Could you check a few things on this model? Use its own coordinates, in mm. A direction names the side the tool comes from. Round coordinates to 2 decimals unless told otherwise and drop trailing zeros. Loops run counter-clockwise (first coordinate to the right, second up) from the corner with the lowest first, then second, coordinate; pieces in that order, holes last. Notation, with made-up numbers: (61, -23.5) - (99, -23.5) arc R19 ccw to (99, -8.5) - close; hole circle Ø11 at (84.25, 56.5). An arc over 180 degrees is marked (long way). Use one line per item in the form item = value.
Autodesk Fusion 360 part; units mm, degrees
sketch "Sketch1" plane through (0, 0, 0) normal (0, 0, 1) x (1, 0, 0)
  line L0 (0, 26.67) -> (-38.1, 26.67)
  line L1 (0, -26.67) -> (-38.1, -26.67)
  line L2 (-38.1, 24.257) -> (0, 24.257)
  line L3 (-38.1, -24.257) -> (0, -24.257)
  line L4 (-38.1, 26.67) -> (-38.1, 24.257)
  line L5 (-38.1, -24.257) -> (-38.1, -26.67)
  arc A0 (0, -26.67) -> (0, 26.67) centre (0, 0) ccw
  arc A1 (0, -24.257) -> (0, 24.257) centre (0, 0) ccw
  dimension "d1" = 53.34
  dimension "d2" = 48.514
  dimension "d3" = 38.1
  dimension "d4" = 38.1
extrude "Extrude1" add sketch "Sketch1" along normal blind 5
sketch "Sketch2" plane through (0, 0, 5) normal (0, 0, 1) x (-1, 0, 0)
  line L0 (38.1, 24.257) -> (38.1, 26.67)
  line L1 (38.1, 26.67) -> (0, 26.67)
  arc A0 (0, 26.67) -> (0, -26.67) centre (0, 0) ccw
  line L2 (0, -26.67) -> (38.1, -26.67)
  line L3 (38.1, -26.67) -> (38.1, -24.257)
  line L4 (38.1, -24.257) -> (0, -24.257)
  arc A1 (0, 24.257) -> (0, -24.257) centre (0, 0) ccw
  line L5 (0, 24.257) -> (38.1, 24.257)
  line L6 (38.1, -26.67) -> (38.1, 26.67)
extrude "Extrude2" add sketch "Sketch2" along normal blind 2.54
sketch "Sketch3" plane through (0, 0, 7.54) normal (0, 0, 1) x (-1, 0, 0)
  line L0 (38.1, -26.67) -> (38.1, 26.67)
  line L1 (38.1, 26.67) -> (0, 26.67)
  arc A0 (0, 26.67) -> (0, -26.67) centre (0, 0) ccw
  line L2 (0, -26.67) -> (38.1, -26.67)
  circle A1 centre (0, 0) radius 16.51
  dimension "d9" = 33.02
extrude "Extrude3" cut sketch "Sketch3" against normal through all contours A1
sketch "Sketch4" plane through (0, 0, 5) normal (0, 0, -1) x (1, 0, 0)
  circle A0 centre (0, 0) radius 16.51
  line L0 (0, 24.257) -> (-38.1, 24.257)
  line L1 (-38.1, 24.257) -> (-38.1, -24.257)
  line L2 (-38.1, -24.257) -> (0, -24.257)
  arc A1 (0, -24.257) -> (0, 24.257) centre (0, 0) ccw
  line L3 (-38.1, 19.257) -> (-35.56, 19.257)
  line L4 (-35.56, 19.257) -> (-35.56, -19.257)
  line L5 (-35.56, -19.257) -> (-38.1, -19.257)
  line L6 (-38.1, -19.257) -> (-38.1, 19.257)
  dimension "d11" = 5
  dimension "d12" = 5
extrude "Extrude4" add sketch "Sketch4" along normal blind 5 contours L1 L3 L4 L5 L6
sketch "Sketch5" plane through (0, 0, 0) normal (0, 0, 1) x (1, 0, 0)
  line L0 (0, 0) -> (30.48, 30.48) construction
  line L1 (0, 0) -> (43.1052, 0) construction
  line L2 (0, 0) -> (33.4313, -33.4313) construction
  line L3 (0, 0) -> (47.279, 0) construction
  circle A0 centre (20.6546, 20.6546) radius 1.4
  circle A1 centre (20.6546, -20.6546) radius 1.4
  circle A2 centre (20.6546, 20.6546) radius 3.175
  line L4 (19.3121, 23.5318) -> (15.3534, 21.8074)
  line L5 (23.5318, 19.3121) -> (21.8074, 15.3534)
  arc A3 (0, -26.67) -> (0, 26.67) centre (0, 0) ccw
  dimension "d15" = 45
  dimension "d16" = 45
  dimension "d17" = 2.8
  dimension "d18" = 2.8
  dimension "d19" = 29.21
  dimension "d20" = 29.21
  dimension "d21" = 6.35
  dimension "d22" = 4.318
extrude "Extrude5" add sketch "Sketch5" along normal blind 3 contours A2 A3 | A2 L4 A3 | A2 L5 A3 picked at (18.4077, 19.9432)
mirror "Mirror1" about plane through (0, 0, 0) normal (0, 1, 0) of "Extrude5"
sketch "Sketch6" plane through (0, 0, 0) normal (0, 0, 1) x (1, 0, 0)
  circle A0 centre (-34.29, -29.21) radius 1.4
  line L0 (-38.1, 26.67) -> (-38.1, -26.67)
  line L1 (-38.1, -26.67) -> (0, -26.67)
  circle A1 centre (-34.29, -29.21) radius 3.175
  line L2 (-37.444, -29.5746) -> (-38.1, -26.67)
  line L3 (-31.136, -29.5746) -> (-30.48, -26.67)
  dimension "d27" = 2.8
  dimension "d28" = 3.81
  dimension "d29" = 2.54
  dimension "d30" = 6.35
extrude "Extrude6" add sketch "Sketch6" along normal blind 3 contours L1 A1 L2 | L1 A1 | L1 A1 L3 picked at (-34.3249, -27.0513)
mirror "Mirror2" about plane through (0, 0, 0) normal (0, 1, 0) of "Extrude6"
sketch "Sketch7" plane through (0, 0, 0) normal (0, 0, 1) x (1, 0, 0)
  line L0 (38.1, -38.1) -> (-38.1, -38.1) construction
  line L1 (-38.1, -38.1) -> (-38.1, 38.1) construction
  line L2 (-38.1, 38.1) -> (38.1, 38.1) construction
  line L3 (38.1, 38.1) -> (38.1, -38.1) construction
  line L4 (38.1, -38.1) -> (-38.1, 38.1) construction
  line L5 (-38.1, -38.1) -> (38.1, 38.1) construction
  dimension "d35" = 76.2
  dimension "d36" = 76.2
1. On a 3-axis mill with a long thin cutter (end or side, diameter ignored), from which of +Z, -Z, +X, -X, +Y, -Y can I reach the whole of each face in a straight line? I mean faces 1 (the face through (-35.56, 0, 3)), 2 (the face through (-19, -24.257, 2)), 3 (the face through (-19, 26.67, 4)), 4 (the face through (21, -19, 3)). Say none if no direction works.
Solution:
face_1 = -Z
face_2 = -Z, -X
face_3 = +Z, +X, +Y
face_4 = +Z, +X, -Y
2. If we section it at D-D, the plane x = 3: Write out the boundary of the cut face in (y, z), plus the area to 3 significant figures.
Solution:
outline = (-26.5, 0) - (-24.07, 0) - (-24.07, 5) - (-16.24, 5) - (-16.24, 7.54) - (-26.5, 7.54) - close; (16.24, 5) - (24.07, 5) - (24.07, 0) - (26.5, 0) - (26.5, 7.54) - (16.24, 7.54) - close
area = 76.4 mm^2
3. If we section it at C-C, the plane z = 6.25: Write out the boundary of the cut face in (x, y), plus the area to 3 significant figures.
Solution:
outline = (-38.1, -26.67) - (0, -26.67) arc R26.67 ccw to (0, 26.67) - (-38.1, 26.67) - close; hole circle Ø33.02 at (0, 0)
area = 2,290 mm^2
4. Please list where these lines run through material, in increasing order: line 1 along Y through (x, z) = (-19, 0.5); line 2 along Z through (x, y) = (18.5, -7); line 3 along Y through (x, z) = (0, 6.1).
Solution:
line_1 = -26.67 to -24.26, 24.26 to 26.67
line_2 = 5 to 7.54
line_3 = -26.67 to -16.51, 16.51 to 26.67
5. If we section it at B-B, the plane y = 3: Write out the boundary of the cut face in (x, z).
Solution:
outline = (-38.1, 0) - (-35.56, 0) - (-35.56, 5) - (-16.24, 5) - (-16.24, 7.54) - (-38.1, 7.54) - close; (16.24, 5) - (24.07, 5) - (24.07, 0) - (26.5, 0) - (26.5, 7.54) - (16.24, 7.54) - close
6. For P1, Ø9.5, axis at x = 20.5, y = 20.5, coming from the +Z side; P2, Ø1.7, axis at x = -35.5, y = 28.5, coming from the +Z side; P3, Ø1.3, axis at x = -36.5, z = 3, coming from the -Y side; P4, Ø4, axis at y = 4.5, z = 2.5, coming from the +X side, each with a flat end and sliding along its axis, tell me the tip position at first contact or that it passes through.
Solution:
P1 = 7.54
P2 = 3
P3 = -31.98
P4 = 26.55
7. If we section it at A-A, the plane x = -34.29: Write out the boundary of the cut face in (y, z) (3 decimals).
Solution:
outline = (-32.385, 0) - (-30.61, 0) - (-30.61, 3) - (-32.385, 3) - close; (-27.81, 0) - (-24.257, 0) - (-24.257, 5) - (24.257, 5) - (24.257, 0) - (27.81, 0) - (27.81, 3) - (26.67, 3) - (26.67, 7.54) - (-26.67, 7.54) - (-26.67, 3) - (-27.81, 3) - close; (30.61, 0) - (32.385, 0) - (32.385, 3) - (30.61, 3) - close
8. We'd pull the mould along X, two halves only. Please class faces 5 (the face through (17.31, -22.66, 1.48)), 6 (the face through (-30.803, 28.102, 1.479)), 7 (the face through (-19, -26.67, 4)): +X half, -X half, draft (parallel to the pull), parting line (faces both ways), or undercut.
Solution:
face_5 = undercut
face_6 = +X half
face_7 = draft
